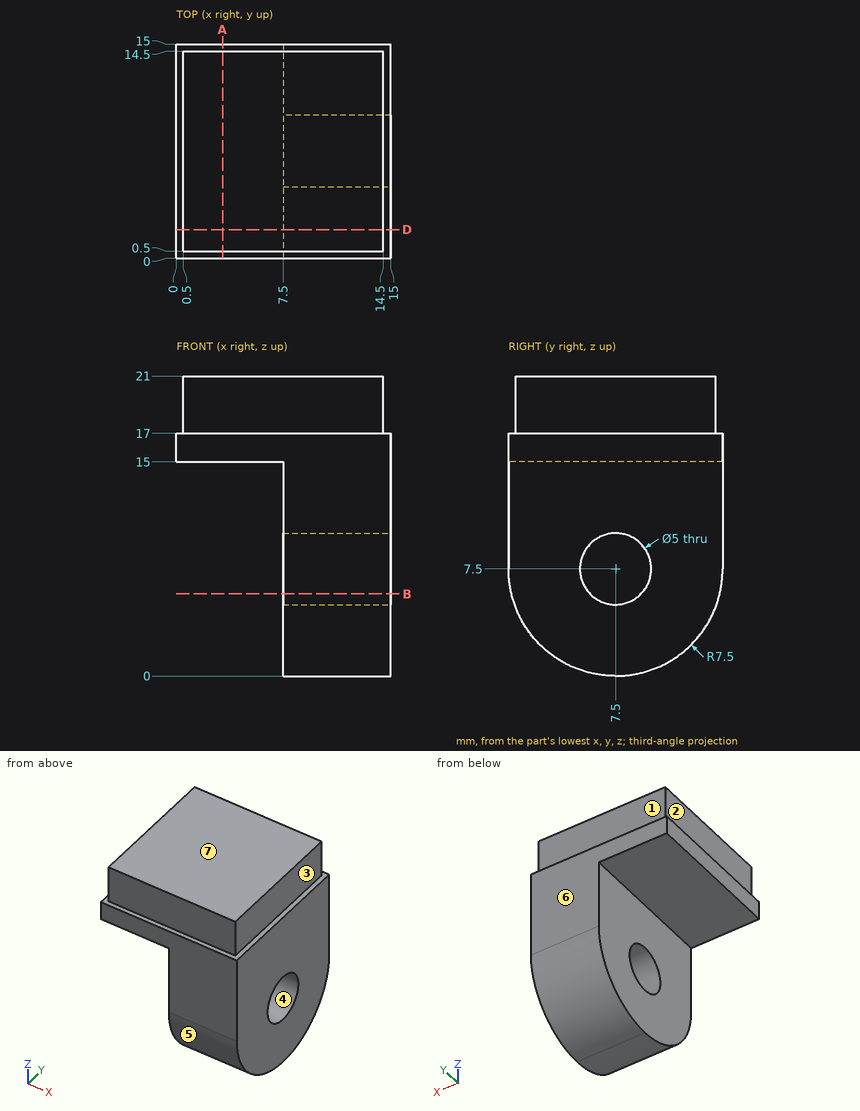
Verification items for this drawing (mm, ordinates from the low corner). A direction names the side the tool comes from. Coordinates: 2 decimals unless noted, no trailing zeros. Loops run counter-clockwise (first coordinate to the right, second up) from the corner with the lowest first, then second, coordinate; pieces in that order, holes last. Notation, with made-up numbers: (43.25, 15) -> (77.25, 15) arc R30 ccw to (77.25, 44) -> close; hole circle Ø2 at (50.5, -12.75). An arc over 180 degrees is marked (long way). Put each result on its own line as item: value.
1. Mould release check, pull along Y, two halves, no side actions. Record for the marked faces 4, 5, 6 and 7: pulls with the +Y half, pulls with the -Y half, needs draft (parallel to the pull), parting line crosses it, or undercut.
Result set:
face 4: undercut
face 5: pulls with the -Y half
face 6: pulls with the +Y half
face 7: needs draft
2. Tool access check on the marked faces 1, 2 and 3. Record the directions out of +Z, -Z, +X, -X, +Y, -Y that give a thin tool (end or side, any length) a straight path to the whole face; none if there is none.
Result set:
face 1: +Z, +X, -X, +Y
face 2: +Z, -X, +Y, -Y
face 3: +Z, +X, +Y, -Y
3. Section check A-A, the plane x = 3.25. Record the boundary of the cut face in (y, z), then the cut area to 3 significant figures.
Result set:
outline: (0, 15) -> (15, 15) -> (15, 17) -> (14.5, 17) -> (14.5, 21) -> (0.5, 21) -> (0.5, 17) -> (0, 17) -> close
area: 86.0 mm^2
4. Thickness scan on line 1 (Z direction, x = 9.25, y = 7.5); line 2 (Z direction, x = 3, y = 4.75); line 3 (X direction, y = 3, z = 8.25). Record the ranges inside material, lowest first.
Result set:
line 1: z = 0 to 5, 10 to 21
line 2: z = 15 to 21
line 3: x = 7.5 to 15
5. Section check B-B, the plane z = 5.75. Record the boundary of the cut face in (x, y).
Result set:
outline: (7.5, 0.21) -> (15, 0.21) -> (15, 5.71) -> (7.5, 5.71) -> close; (7.5, 9.29) -> (15, 9.29) -> (15, 14.79) -> (7.5, 14.79) -> close
6. Gauge pin test, flat ends, axial feed: P1, Ø4.5, axis at x = 9, z = 19, coming from the +Y side; P2, Ø5, axis at x = 12, y = 4, coming from the -Z side; P3, Ø1.2, axis at y = 10, z = 18, coming from the -X side; P4, Ø2, axis at y = 9, z = 10, coming from the -X side. Record the tip position at first contact, or that the pin passes through.
Result set:
P1: stops at y = 15
P2: stops at z = 0.07
P3: stops at x = 0.5
P4: stops at x = 7.5
7. Section check D-D, the plane y = 2. Record the boundary of the cut face in (x, z), then the cut area to 3 significant figures.
Result set:
outline: (0, 15) -> (7.5, 15) -> (7.5, 2.4) -> (15, 2.4) -> (15, 17) -> (14.5, 17) -> (14.5, 21) -> (0.5, 21) -> (0.5, 17) -> (0, 17) -> close
area: 180 mm^2
